from build123d import *

# Parameters (mm, degrees)
BOSS_EXTRUDE2_DEPTH = 10
CUT_EXTRUDE3_DEPTH  = 1.6
SKETCH5_W           = 8.164929968
SKETCH5_H           = 9.761243885
CUT_EXTRUDE4_DEPTH  = 19.6
SKETCH6_R           = 1
CUT_EXTRUDE5_DEPTH  = 5


with BuildPart() as part:
    # Sketch2 → Boss-Extrude2 (new body)
    with BuildSketch(Plane.XY):
        with BuildLine():
            Line((-9.5, 6), (9.5, 6))
            ThreePointArc((9.5, 6), (10.207106781, 5.707106781), (10.5, 5))
            Line((10.5, 5), (10.5, -5))
            ThreePointArc((10.5, -5), (10.207106781, -5.707106781), (9.5, -6))
            Line((9.5, -6), (-9.5, -6))
            ThreePointArc((-9.5, -6), (-10.207106781, -5.707106781), (-10.5, -5))
            Line((-10.5, -5), (-10.5, 5))
            ThreePointArc((-10.5, 5), (-10.207106781, 5.707106781), (-9.5, 6))
        make_face()
    extrude(amount=BOSS_EXTRUDE2_DEPTH)

    # Sketch4 → Cut-Extrude3 (cut)
    with BuildSketch(Plane(origin=(0, 0, 0), x_dir=(-1, 0, 0), z_dir=(0, 0, -1))):
        with BuildLine():
            Line((-9.759787833, 5.35287298), (9.740212167, 5.35287298))
            ThreePointArc((9.740212167, 5.35287298), (9.810922845, 5.323583659), (9.840212167, 5.25287298))
            Line((9.840212167, 5.25287298), (9.840212167, -5.296629435))
            ThreePointArc((9.840212167, -5.296629435), (9.810922845, -5.367340113), (9.740212167, -5.396629435))
            Line((9.740212167, -5.396629435), (-9.759787833, -5.396629435))
            ThreePointArc((-9.759787833, -5.396629435), (-9.830498511, -5.367340113), (-9.859787833, -5.296629435))
            Line((-9.859787833, -5.296629435), (-9.859787833, 5.25287298))
            ThreePointArc((-9.859787833, 5.25287298), (-9.830498511, 5.323583659), (-9.759787833, 5.35287298))
        make_face()
    extrude(amount=-CUT_EXTRUDE3_DEPTH, mode=Mode.SUBTRACT)

    # Sketch5 → Cut-Extrude4 (cut)
    with BuildSketch(Plane.ZY.offset(9.8)):
        with Locations((5.717262672, 0.005392953)):
            Rectangle(SKETCH5_W, SKETCH5_H)
    extrude(amount=-CUT_EXTRUDE4_DEPTH, mode=Mode.SUBTRACT)

    # Sketch6 → Cut-Extrude5 (cut)
    with BuildSketch(Plane.XZ.offset(6)):
        with Locations(Location((0, 5, 0), (0, 0, 270))):
            Circle(SKETCH6_R)
    extrude(amount=-CUT_EXTRUDE5_DEPTH, mode=Mode.SUBTRACT)


solid = part.part
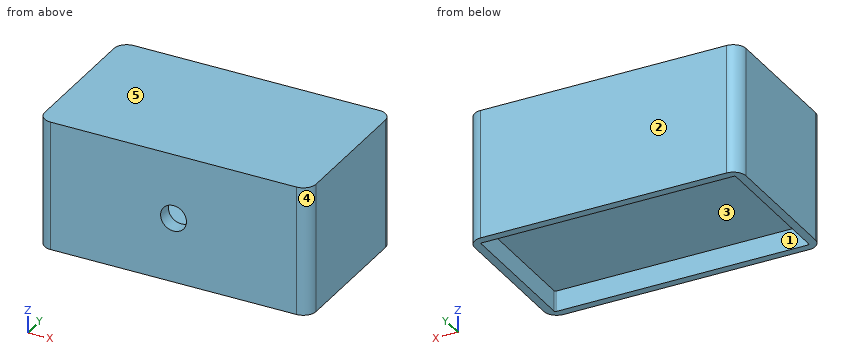
CAD build for the part. Positions are in the model's coordinates, mm. Face numbers are marked on the shaded views. A direction names the side the tool comes from. Round coordinates to 2 decimals unless told otherwise and drop trailing zeros. Write each loop counter-clockwise with the first axis right and the second up, starting at its lowest first coordinate (ties: lowest second). Pieces come first, ordered by that corner, then holes.
(1) Slice it at D-D, the plane z = 5. Write the cut outline in (x, y).
(2) Slice it at B-B, the plane z = 8. Write the cut outline in (x, y).
(3) Slice it at A-A, the plane x = 5.5. Write the cut outline in (y, z), and give its area (3 significant figures).
(4) Slice it at C-C, the plane x = 0. Write the cut outline in (y, z).
(5) Drop flat-ended pins along their axis: P1, Ø1, axis at x = -3, y = 2.5, coming from the -Z side; P2, Ø1.8, axis at x = 0, z = 5, coming from the -Y side. Give the stop position or say it passes through.
(6) Probe line 1 along Y through (x, z) = (3, 0.5); line 2 along Y through (x, z) = (1.75, 7); line 3 along X through (y, z) = (2, 7.75). List the from-to ranges inside material, lowest first.
(7) 3-axis set-ups, long thin cutter, end or side, ignore diameter. For the marked faces 1 and 2: which of +Z, -Z, +X, -X, +Y, -Y reach the whole face in a straight line?
(8) Mould opens along Y. For the marked faces 3, 4 and 5 say: pulls with the +Y half, pulls with the -Y half, needs draft (parallel to the pull), parting line crosses it, or undercut.
From the geometry:
1. outline: (-10.5, -5) arc R1 ccw to (-9.5, -6) - (-1, -6) - (-1, -4.88) - (-9.8, -4.88) - (-9.8, 4.89) - (9.8, 4.89) - (9.8, -4.88) - (1, -4.88) - (1, -6) - (9.5, -6) arc R1 ccw to (10.5, -5) - (10.5, 5) arc R1 ccw to (9.5, 6) - (-9.5, 6) arc R1 ccw to (-10.5, 5) - close
2. outline: (-10.5, -5) arc R1 ccw to (-9.5, -6) - (9.5, -6) arc R1 ccw to (10.5, -5) - (10.5, 5) arc R1 ccw to (9.5, 6) - (-9.5, 6) arc R1 ccw to (-10.5, 5) - close; hole (-9.8, -4.88) - (9.8, -4.88) - (9.8, 4.89) - (-9.8, 4.89) - close
3. outline: (-6, 0) - (-5.4, 0) - (-5.4, 1.6) - (5.35, 1.6) - (5.35, 0) - (6, 0) - (6, 10) - (-6, 10) - close; hole (-4.88, 1.63) - (4.89, 1.63) - (4.89, 9.8) - (-4.88, 9.8) - close
3. area: 23.1 mm2
4. outline: (-6, 0) - (-5.4, 0) - (-5.4, 1.6) - (5.35, 1.6) - (5.35, 0) - (6, 0) - (6, 10) - (-6, 10) - (-6, 6) - (-4.88, 6) - (-4.88, 9.8) - (4.89, 9.8) - (4.89, 1.63) - (-4.88, 1.63) - (-4.88, 4) - (-6, 4) - close
5. P1: stops at z = 1.6
5. P2: stops at y = 4.89
6. line 1: y = -6 to -5.4, 5.35 to 6
6. line 2: y = -6 to -4.88, 4.89 to 6
6. line 3: x = -10.5 to -9.8, 9.8 to 10.5
7. face 1: -Z
7. face 2: +Z, -Z, +X, -X, +Y
8. face 3: undercut
8. face 4: pulls with the -Y half
8. face 5: needs draft
